Here's how the part is built. I have some questions about the finished solid (model axes, mm). Face numbers are marked on the shaded views. A direction names the side the tool comes from. Coordinates: 2 decimals unless noted, no trailing zeros. Write each loop counter-clockwise with the first axis right and the second up, starting at its lowest first coordinate (ties: lowest second). Pieces come first, ordered by that corner, then holes.
from build123d import *

# Parameters (mm, degrees)
BOSS_EXTRUDE1_DEPTH = 10
SKETCH6_W           = 20
SKETCH6_H           = 5
BOSS_EXTRUDE2_DEPTH = 20.1
SKETCH8_W           = 5.5
SKETCH8_H           = 15
CUT_EXTRUDE1_DEPTH  = 20
SKETCH9_R           = 2.05
CUT_EXTRUDE2_DEPTH  = 50
SKETCH2_R           = 2
CUT_EXTRUDE3_DEPTH  = 10
MIRROR3_OUTLINE_R   = 2
MIRROR3_DEPTH       = 10


# Read off the part's stored shape, not the designer's step: Mirror3
with BuildPart() as part:
    # Sketch1 → Boss-Extrude1 (new body)
    with BuildSketch(Plane.XY):
        Polygon((0, 0), (0, 23), (29.5, 23), (39.5, 20), (49.5, 20), (49.5, 15), (29.5, 15), (29.5, 5), (49.5, 5), (49.5, 0), align=None)
    extrude(amount=BOSS_EXTRUDE1_DEPTH)

    # Sketch6 → Boss-Extrude2 (add)
    with BuildSketch(Plane(origin=(0, 0, 0), x_dir=(-1, 0, 0), z_dir=(0, 0, -1))):
        Polygon((-29.5, 15), (-49.5, 15), (-49.5, 20), (-39.5, 20), (-29.5, 23), (0, 23), (0, 20), (-29.5, 20), align=None)
        with Locations((-39.5, 2.5)):
            Rectangle(SKETCH6_W, SKETCH6_H)
    extrude(amount=BOSS_EXTRUDE2_DEPTH)

    # Mirror2: part across face


with BuildPart() as part_1:
    add(part.part)
    add(part.part.mirror(Plane(origin=(28.245085995, 19.497542998, -20.1), x_dir=(1, 0, 0), z_dir=(0, 0, -1))))

    # Sketch8 → Cut-Extrude1 (cut)
    with BuildSketch(Plane.XY.offset(10)):
        with Locations((21.75, 7.5)):
            Rectangle(SKETCH8_W, SKETCH8_H)
    extrude(amount=-CUT_EXTRUDE1_DEPTH, mode=Mode.SUBTRACT)

    # Sketch9 → Cut-Extrude2 (cut)
    with BuildSketch(Plane.XZ):
        with Locations(Location((44.5, -3, 0), (0, 0, 270))):
            Circle(SKETCH9_R)
        with Locations(Location((44.5, -45.2, 0), (0, 0, 270))):
            Circle(SKETCH9_R)
        with Locations(Location((44.5, -20, 0), (0, 0, 270))):
            Circle(SKETCH9_R)
    extrude(amount=-CUT_EXTRUDE2_DEPTH, mode=Mode.SUBTRACT)

    # Sketch2 → Cut-Extrude3 (cut)
    with BuildSketch(Plane.ZY):
        with Locations((3.9, 5)):
            Circle(SKETCH2_R)
        with Locations((3.9, 15)):
            Circle(SKETCH2_R)
    extrude(amount=-CUT_EXTRUDE3_DEPTH, mode=Mode.SUBTRACT)

    # Mirror3 outline → Mirror3 (cut)
    with BuildSketch(Plane.YZ):
        with Locations((15, -44.1)):
            Circle(MIRROR3_OUTLINE_R)
        with Locations((5, -44.1)):
            Circle(MIRROR3_OUTLINE_R)
    extrude(amount=MIRROR3_DEPTH, mode=Mode.SUBTRACT)


solid = part_1.part
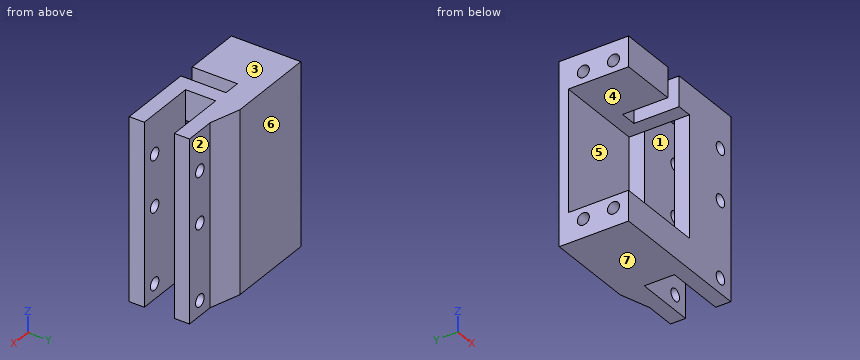
1. I want a section at B-B (z = -12.5). List the corners of the cut face in (x, y) for me.
2. I want a section at C-C (x = 35). List the corners of the cut face in (y, z) for me.
3. I want a section at D-D (y = 8.5). List the corners of the cut face in (x, z) for me, then the cut area to 3 significant figures.
4. For pin 1 Ø1.6 at (x, z) = (21, 6) entering from -Y; pin 2 Ø6 at (x, z) = (35.5, -24) entering from +Y; pin 3 Ø5.5 at (x, z) = (44.5, -20) entering from +Y, each with a flat end and sliding along its axis, tell me the tip position at first contact or that it passes through.
5. Thinking about a two-plate mould opening in Z: for the marked faces 4, 5, 6 and 7, which applies, pulls with the +Z half, pulls with the -Z half, needs draft (parallel to the pull), parting line crosses it, or undercut?
6. I want a section at A-A (x = 44.5). State how many separate pieces and enclosed holes the cut face has, then the cut area to 3 significant figures.
7. On a 3-axis mill with a long thin cutter (end or side, diameter ignored), from which of +Z, -Z, +X, -X, +Y, -Y can I reach the whole of each face in a straight line? I mean the marked faces 1, 2 and 3. Say none if no direction works.
8. If I drill on line 1 (Y direction, x = 6, z = -44); line 2 (Z direction, x = 11, y = 16.25); line 3 (Y direction, x = 44.5, z = -25), over which ranges is the centre line in solid material (lowest first)?
Response values:
1. outline: (0, 20) - (29.5, 20) - (29.5, 15) - (49.5, 15) - (49.5, 20) - (39.5, 20) - (29.5, 23) - (0, 23) - close; (29.5, 0) - (49.5, 0) - (49.5, 5) - (29.5, 5) - close
2. outline: (0, -50.2) - (5, -50.2) - (5, 10) - (0, 10) - close; (15, -50.2) - (21.35, -50.2) - (21.35, 10) - (15, 10) - close
3. outline: (0, -50.2) - (29.5, -50.2) - (29.5, -40.2) - (0, -40.2) - close; (0, 0) - (19, 0) - (19, 10) - (0, 10) - close; (24.5, 0) - (29.5, 0) - (29.5, 10) - (24.5, 10) - close
3. area: 535 mm2
4. pin 1: stops at y = 15
4. pin 2: stops at y = 22.1
4. pin 3: stops at y = 20
5. face 4: undercut
5. face 5: undercut
5. face 6: needs draft
5. face 7: pulls with the -Z half
6. separate pieces: 8
6. enclosed holes: 0
6. area: 479 mm2
7. face 1: +Z, -Z, +X
7. face 2: +Z, -Z, +X, +Y
7. face 3: +Z, +X, -X, +Y, -Y
8. line 1: y = 0 to 3, 7 to 13, 17 to 23
8. line 2: z = -50.2 to -40.2, 0 to 10
8. line 3: y = 0 to 5, 15 to 20
